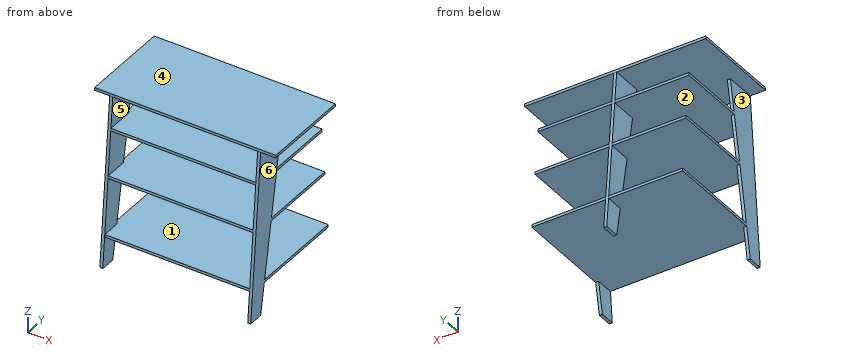
```python
from build123d import *

# Parameters (mm, degrees)
F0_W     = 600
F0_H     = 18
F1_DEPTH = 600
F4_DEPTH = 20
F6_DEPTH = 10
F7_W     = 691.8869644485
F7_H     = 18
F7_W_2   = 636.4630811304
F7_W_3   = 760.2552415679
F8_DEPTH = 500


with BuildPart() as f1:
    # F0 (on Front) → F1 (new body)
    with BuildSketch(Plane.XZ):
        with Locations((-300, 1106)):
            Rectangle(F0_W, F0_H)
    extrude(amount=F1_DEPTH)

    # F3 (on offset) → F4 (join)
    with BuildSketch(Plane.YZ.offset(-500)):
        Polygon((-600, 0), (-400, 1097), (-600, 1097), (-700, 0), align=None)
    extrude(amount=F4_DEPTH)

    # F5 (on Right) → F6 (join)
    with BuildSketch(Plane.YZ):
        Polygon((100, 0), (0, 1097), (-200, 1097), (0, 0), align=None)
    extrude(amount=-F6_DEPTH)

    # F7 (on offset) → F8 (join)
    with BuildSketch(Plane.YZ.offset(-500)):
        with Locations((-300, 584)):
            Rectangle(F7_W, F7_H)
        with Locations((-300, 888)):
            Rectangle(F7_W_2, F7_H)
        with Locations((-300, 209)):
            Rectangle(F7_W_3, F7_H)
    extrude(amount=F8_DEPTH)

    # F9: F1 across plane


with BuildPart() as f1_1:
    add(f1.part)
    add(f1.part.mirror(Plane.YZ))


solid = f1_1.part
```
Read the model definition and answer for the solid it produces. Units are mm, in the model's axes. Face numbers are marked on the shaded views. A direction names the side the tool comes from. Coordinates: 2 decimals unless noted, no trailing zeros. Loops run counter-clockwise (first coordinate to the right, second up) from the corner with the lowest first, then second, coordinate; pieces in that order, holes last.
(1) A tool of negligible diameter and unlimited length cuts with its end or side. For the marked faces 5 and 6, from which of +Z, -Z, +X, -X, +Y, -Y can it reach the whole face along a straight path? Write none if from no direction.
Solution:
face 5: +Y, -Y
face 6: -Z, +X, +Y, -Y
(2) The part is cut by section A-A (x = -235.5). Determine the outline of the cut face in (y, z), and give its area (3 significant figures).
Solution:
outline: (-680.13, 200) - (80.13, 200) - (80.13, 218) - (-680.13, 218) - close; (-645.94, 575) - (45.94, 575) - (45.94, 593) - (-645.94, 593) - close; (-618.23, 879) - (18.23, 879) - (18.23, 897) - (-618.23, 897) - close; (-600, 1097) - (0, 1097) - (0, 1115) - (-600, 1115) - close
area: 48,400 mm2
(3) The part is cut by section C-C (y = -528). Determine the outline of the cut face in (x, z), and give its area (3 significant figures).
Solution:
outline: (-600, 1097) - (-500, 1097) - (-500, 394.92) - (-480, 394.92) - (-480, 575) - (480, 575) - (480, 394.92) - (500, 394.92) - (500, 1097) - (600, 1097) - (600, 1115) - (-600, 1115) - close; (-500, 200) - (500, 200) - (500, 218) - (-500, 218) - close; hole (-480, 593) - (480, 593) - (480, 879) - (-480, 879) - close; hole (-480, 897) - (480, 897) - (480, 1097) - (-480, 1097) - close
area: 102,000 mm2
(4) The part is cut by section B-B (y = -304). Determine the outline of the cut face in (x, z), and give its area (3 significant figures).
Solution:
outline: (-600, 1097) - (600, 1097) - (600, 1115) - (-600, 1115) - close; (-500, 200) - (500, 200) - (500, 218) - (-500, 218) - close; (-500, 575) - (500, 575) - (500, 593) - (-500, 593) - close; (-500, 879) - (500, 879) - (500, 897) - (-500, 897) - close
area: 75,600 mm2
(5) Flat-ended cylindrical pins translate along their axes: pin 1 Ø14.5 at (x, z) = (-260.5, 1106.5) entering from +Y; pin 2 Ø5.5 at (x, z) = (308, 891.5) entering from +Y; pin 3 Ø14.5 at (x, z) = (209, 212) entering from +Y. Find the tip coordinate at first contact, or state that the pin passes through.
Solution:
pin 1: stops at y = 0
pin 2: stops at y = 18.23
pin 3: stops at y = 80.13
(6) Consider line 1 along Z through (x, y) = (-104, -497.5); line 2 along Z through (x, y) = (467, 9.5); line 3 along Z through (x, y) = (297.5, 40.5). Determine where each line is inside the solid, lowest interval first.
Solution:
line 1: z = 200 to 218, 575 to 593, 879 to 897, 1097 to 1115
line 2: z = 200 to 218, 575 to 593, 879 to 897
line 3: z = 200 to 218, 575 to 593
(7) The mould has two halves that part along Z. Classify the marked faces 1, 2, 3 and 4: released by +Z, released by -Z, zero draft, split by the parting line, or undercut.
Solution:
face 1: undercut
face 2: undercut
face 3: zero draft
face 4: released by +Z
(8) The part is cut by section D-D (z = 615.5). Determine the outline of the cut face in (x, y), and give its area (3 significant figures).
Solution:
outline: (-500, -643.89) - (-480, -643.89) - (-480, -487.78) - (-500, -487.78) - close; (-10, -112.22) - (10, -112.22) - (10, 43.89) - (-10, 43.89) - close; (480, -643.89) - (500, -643.89) - (500, -487.78) - (480, -487.78) - close
area: 9,370 mm2
